from build123d import *

# Parameters (mm, degrees)
CHAMFER1_SIZE           = 0.5
SKETCH2_R               = 2.5
CUT_EXTRUDE1_DEPTH      = 1
CUT_EXTRUDE1_DEPTH_BACK = 17


with BuildPart() as part:
    # Sketch1 → Revolve1 (revolve)
    with BuildSketch(Plane.XY):
        Polygon((-6, 8), (-6, -8), (-21, -8), (-21, -5), (-10, -5), (-10, 5), (-21, 5), (-21, 8), align=None)
    revolve(axis=Axis((0, 39.685139112, 0), (0, -1, 0)))

    # Chamfer1
    chamfer1_edges = [part.edges().sort_by_distance(p)[0] for p in [
        (21, -8, 0),
        (21, 8, 0),
        (21, 5, 0),
        (21, -5, 0),
    ]]
    chamfer(chamfer1_edges, length=CHAMFER1_SIZE)

    # Sketch2 → Cut-Extrude1 (cut, two sides)
    with BuildSketch(Plane.XZ.offset(8)) as cut_extrude1_sk:
        with Locations((0, 16)):
            Circle(SKETCH2_R)
        with Locations((13.856406461, 8)):
            Circle(SKETCH2_R)
        with Locations((13.856406461, -8)):
            Circle(SKETCH2_R)
        with Locations((0, -16)):
            Circle(SKETCH2_R)
        with Locations((-13.856406461, -8)):
            Circle(SKETCH2_R)
        with Locations((-13.856406461, 8)):
            Circle(SKETCH2_R)
    extrude(amount=CUT_EXTRUDE1_DEPTH, mode=Mode.SUBTRACT)
    extrude(cut_extrude1_sk.sketch, amount=-CUT_EXTRUDE1_DEPTH_BACK, mode=Mode.SUBTRACT)


solid = part.part
Check sheet for the modelled part. Datum: model origin and axes. Units: mm. A direction names the side the tool comes from. Round coordinates to 2 decimals unless told otherwise and drop trailing zeros. Order: outer loops, then holes, each group sorted by start corner. A loop starts at its lowest first (then second) coordinate and runs counter-clockwise, first axis right, second up. Notation, with made-up numbers: M -28,18.25 L 9,18.25 A14 ccw 9,34.25 Z; hole C 38.25,-6 d10. An arc over 180 degrees is marked long. One line per item, written item: value. Start each with the question number.
1. Gauge pin test, flat ends, axial feed: P1, Ø9.5, axis at x = 0, z = 0, coming from the -Y side; P2, Ø1, axis at y = -1.5, z = 8, coming from the -X side; P3, Ø8, axis at y = 2, z = 11, coming from the +X side; P4, Ø1.5, axis at y = -6.5, z = 2.5, coming from the -X side. Record the tip position at first contact, or that the pin passes through.
2. Release check for a two-part mould opening along X. For faces 1 (the flat face through (9, 5, -5)), 2 (the cylindrical face through (11.87, 6.48, -9.52)), 3 (the cylindrical face through (-15.84, 6.48, 6.48)), 4 (the cylindrical face through (-20.03, 6.51, -6.31)) record: released by +X, released by -X, zero draft, split by the parting line, or undercut.
3. Section check C-C on y = -4.5. Enter the section's corners in (x, z), and give its area (3 significant figures).
4. Scan lines: line 1 along Z through (x, y) = (0, 7.1); line 2 along Y through (x, z) = (-15, 4); line 3 along Z through (x, y) = (-12.5, 5.25). Record each from-to range of solid material in increasing order.
5. Access from +Z, -Z, +X, -X, +Y, -Y to the whole of each face (thin tool, end or side, straight path). Record for faces 5 (the cylindrical face through (11.87, 6.48, 6.48)), 6 (the flat face through (-9, -5, -5)).
6. Section check A-A on z = 0. Enter the section's corners in (x, y).
7. Section check B-B on x = 0. Give the number of separate pieces and of enclosed holes in the cut face, and give its area (3 significant figures).
Results found:
1. P1: through
1. P2: x = -6.61
1. P3: x = 18.94
1. P4: x = -20.93
2. face 1: zero draft
2. face 2: undercut
2. face 3: undercut
2. face 4: split by the parting line
3. outline: C 0,0 d20; hole C 0,0 d12
3. area: 201 mm^2
4. line 1: -21 to -18.5, -13.5 to -6, 6 to 13.5, 18.5 to 21
4. line 2: -8 to -5, 5 to 8
4. line 3: -16.56 to -10.1, -5.9 to 5.9, 10.1 to 16.56
5. face 5: +Y, -Y
5. face 6: none
6. outline: M -21,-7.5 L -20.5,-8 L -6,-8 L -6,8 L -20.5,8 L -21,7.5 L -21,5.5 L -20.5,5 L -10,5 L -10,-5 L -20.5,-5 L -21,-5.5 Z; M 6,-8 L 20.5,-8 L 21,-7.5 L 21,-5.5 L 20.5,-5 L 10,-5 L 10,5 L 20.5,5 L 21,5.5 L 21,7.5 L 20.5,8 L 6,8 Z
7. separate pieces: 6
7. enclosed holes: 0
7. area: 199 mm^2
